The listing builds one solid part. Answer for the finished solid, in the listing's coordinates (mm). Round coordinates to 2 decimals unless told otherwise and drop trailing zeros. Write each loop counter-clockwise with the first axis right and the second up, starting at its lowest first coordinate (ties: lowest second). Pieces come first, ordered by that corner, then holes. Notation, with made-up numbers: (-12, 39) - (28, 39) arc R14 ccw to (28, 53) - close; hole circle Ø9 at (-24.75, -3). An arc over 180 degrees is marked (long way). Answer as CSV lines item,"result". Start each with the question number.
Item 1: A cutting plane is placed at A-A on x = 24. Determine the outline of the cut face in (y, z).
Item 2: Straight lines are drawn through the part: line 1 along Y through (x, z) = (24, -2); line 2 along Y through (x, z) = (25.25, -4.6); line 3 along X through (y, z) = (-5.5, -4.5). For each, find the intervals that lie inside material, in ascending order. Write a range as [from, to].
Item 3: A cutting plane is placed at C-C on z = -4.3. Determine the outline of the cut face in (x, y), and give its area (3 significant figures).
Item 4: For a pull along Y with two mould halves and no side action, classify faces 1 (the cylindrical face through (22.4, -6.2, -2.5)), 2 (the flat face through (22, 0, -5)), 3 (the cylindrical face through (26.55, 9.07, -2.46)) as pulls with the +Y half, pulls with the -Y half, needs draft (parallel to the pull), parting line crosses it, or undercut.
Item 5: A cutting plane is placed at B-B on y = 5. Determine the outline of the cut face in (x, z).
Item 6: A cutting plane is placed at D-D on x = 22.25. Determine the outline of the cut face in (y, z).
```python
from build123d import *

# Parameters (mm, degrees)
SKETCH1_R           = 2
SKETCH1_R_2         = 1.5
BOSS_EXTRUDE2_DEPTH = 5


with BuildPart() as part:
    # Sketch1 → Boss-Extrude2 (new body)
    with BuildSketch(Plane.XY):
        with BuildLine():
            Line((20, -9.5), (20, 9.5))
            Line((20, 9.5), (25.5, 9.5))
            ThreePointArc((25.5, 9.5), (26.560660172, 9.060660172), (27, 8))
            Line((27, 8), (27, -8))
            ThreePointArc((27, -8), (26.560660172, -9.060660172), (25.5, -9.5))
            Line((25.5, -9.5), (20, -9.5))
        make_face()
        with Locations((24, 5)):
            Circle(SKETCH1_R, mode=Mode.SUBTRACT)
        with Locations((24, -5)):
            Circle(SKETCH1_R, mode=Mode.SUBTRACT)
        with Locations((24, 0)):
            Circle(SKETCH1_R_2, mode=Mode.SUBTRACT)
    extrude(amount=-BOSS_EXTRUDE2_DEPTH)


solid = part.part
```
Geometry says:
1,outline,"(-9.5, -5) - (-7, -5) - (-7, 0) - (-9.5, 0) - close; (-3, -5) - (-1.5, -5) - (-1.5, 0) - (-3, 0) - close; (1.5, -5) - (3, -5) - (3, 0) - (1.5, 0) - close; (7, -5) - (9.5, -5) - (9.5, 0) - (7, 0) - close"
2,line 1,"y = [-9.5, -7], [-3, -1.5], [1.5, 3], [7, 9.5]"
2,line 2,"y = [-9.5, -6.56], [-3.44, -0.83], [0.83, 3.44], [6.56, 9.5]"
2,line 3,"x = [20, 22.06], [25.94, 27]"
3,outline,"(20, -9.5) - (25.5, -9.5) arc R1.5 ccw to (27, -8) - (27, 8) arc R1.5 ccw to (25.5, 9.5) - (20, 9.5) - close; hole circle Ø4 at (24, -5); hole circle Ø4 at (24, 5); hole circle Ø3 at (24, 0)"
3,area,"99.8 mm^2"
4,face 1,"undercut"
4,face 2,"needs draft"
4,face 3,"pulls with the +Y half"
5,outline,"(20, -5) - (22, -5) - (22, 0) - (20, 0) - close; (26, -5) - (27, -5) - (27, 0) - (26, 0) - close"
6,outline,"(-9.5, -5) - (-5.97, -5) - (-5.97, 0) - (-9.5, 0) - close; (-4.03, -5) - (4.03, -5) - (4.03, 0) - (-4.03, 0) - close; (5.97, -5) - (9.5, -5) - (9.5, 0) - (5.97, 0) - close"
